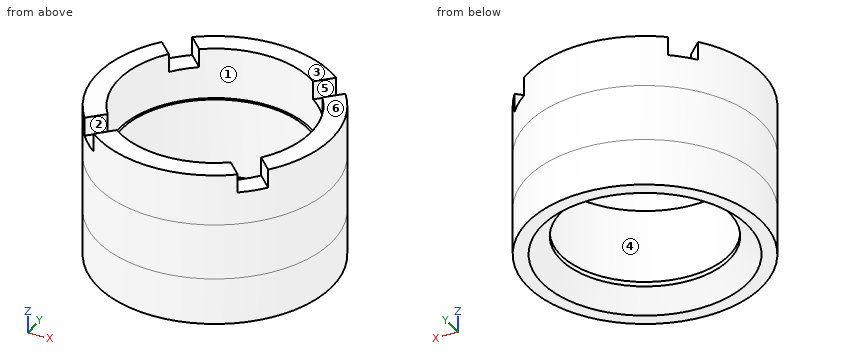
from build123d import *

# Parameters (mm, degrees)
F0_R      = 27
F0_R_2    = 18
F1_DEPTH  = 22
F2_R      = 20
F3_DEPTH  = 17
F4_SIZE   = 4
F5_R      = 27
F5_R_2    = 25
F6_DEPTH  = 12
F7_R      = 25
F7_R_2    = 20.5
F8_DEPTH  = 11
F10_DEPTH = 4
F11_R     = 27
F11_R_2   = 25
F12_DEPTH = 10.001


with BuildPart() as f1:
    # F0 (on Top) → F1 (new body)
    with BuildSketch(Plane.XY):
        Circle(F0_R)
        Circle(F0_R_2, mode=Mode.SUBTRACT)
    extrude(amount=-F1_DEPTH)

    # F2 (on face) → F3 (cut)
    with BuildSketch(Plane.XY):
        Circle(F2_R)
    extrude(amount=-F3_DEPTH, mode=Mode.SUBTRACT)

    # F4
    f4_edges = [f1.edges().sort_by_distance(p)[0] for p in [
        (-18, 0, -22),
    ]]
    chamfer(f4_edges, length=F4_SIZE)

    # F5 (on Top) → F6 (cut)
    with BuildSketch(Plane.XY):
        Circle(F5_R)
        Circle(F5_R_2, mode=Mode.SUBTRACT)
    extrude(amount=-F6_DEPTH, mode=Mode.SUBTRACT)

    # F7 (on face) → F8 (join)
    with BuildSketch(Plane.XY):
        Circle(F7_R)
        Circle(F7_R_2, mode=Mode.SUBTRACT)
    extrude(amount=F8_DEPTH)

    # F9 (on face) → F10 (cut)
    with BuildSketch(Plane.XY.offset(11)):
        Polygon((-28.467241, 32.709882), (-32.709882, 28.467241), (-4.242641, 0), (0, 4.242641), align=None)
        Polygon((0, -4.242641), (-4.242641, 0), (-34.573084, -30.330443), (-30.330443, -34.573084), align=None)
        Polygon((4.242641, 0), (0, -4.242641), (30.929728, -35.172369), (35.172369, -30.929728), align=None)
        Polygon((29.066526, 33.309167), (0, 4.242641), (4.242641, 0), (33.309167, 29.066526), align=None)
    extrude(amount=-F10_DEPTH, mode=Mode.SUBTRACT)

    # F11 (on face) → F12 (cut, through all)
    with BuildSketch(Plane.XY.offset(-12)):
        Circle(F11_R)
        Circle(F11_R_2, mode=Mode.SUBTRACT)
    extrude(amount=-F12_DEPTH, mode=Mode.SUBTRACT)


solid = f1.part
Geometry: final body of the model. Coordinates: model frame, mm. Face numbers are marked on the shaded views. A direction names the side the tool comes from. Round coordinates to 2 decimals unless told otherwise and drop trailing zeros. Order: outer loops, then holes, each group sorted by start corner. A loop starts at its lowest first (then second) coordinate and runs counter-clockwise, first axis right, second up.
Q1. Section D-D, the plane z = -6.5. Output: boundary loops of the cut face in (x, y).
Result sheet:
outline: circle Ø50 at (0, 0); hole circle Ø40 at (0, 0)
Q2. Section C-C, the plane z = 8. Output: boundary loops of the cut face in (x, y), and give its area (3 significant figures).
Result sheet:
outline: (-19.67, -15.43) - (-16.46, -12.22) arc R20.5 cw to (-16.46, 12.22) - (-19.67, 15.43) arc R25 ccw to start; (-15.43, -19.67) arc R25 ccw to (15.43, -19.67) - (12.22, -16.46) arc R20.5 cw to (-12.22, -16.46) - close; (-15.43, 19.67) - (-12.22, 16.46) arc R20.5 cw to (12.22, 16.46) - (15.43, 19.67) arc R25 ccw to start; (16.46, -12.22) - (19.67, -15.43) arc R25 ccw to (19.67, 15.43) - (16.46, 12.22) arc R20.5 cw to start
area: 535 mm2
Q3. Access query for the marked faces 1, 2 and 3. Directions: +Z, -Z, +X, -X, +Y, -Y. A direction counts if a zero-diameter tool reaches every point of the face in a straight line with its end or side. Return the directions, or none.
Result sheet:
face 1: +Z
face 2: +Z, -Y
face 3: +Z, +X, -X, +Y, -Y
Q4. Section A-A, the plane y = 0. Output: boundary loops of the cut face in (x, z), and give its area (3 significant figures).
Result sheet:
outline: (-25, -22) - (-22, -22) - (-18, -18) - (-18, -17) - (-20, -17) - (-20, 0) - (-20.5, 0) - (-20.5, 11) - (-25, 11) - close; (18, -18) - (22, -22) - (25, -22) - (25, 11) - (20.5, 11) - (20.5, 0) - (20, 0) - (20, -17) - (18, -17) - close
area: 323 mm2
Q5. Material intervals for probe 1 along X at (y, z) = (0, 8); probe 2 along Y at (x, z) = (0, -12); probe 3 along Y at (x, z) = (5, -1.5), sorted ascending.
Result sheet:
probe 1: x = -25 to -20.5, 20.5 to 25
probe 2: y = -25 to -20, 20 to 25
probe 3: y = -24.49 to -19.36, 19.36 to 24.49
Q6. Pin query (flat end, axial travel): pin 1 (5 mm diameter, centred on x = -13, z = 2, fed in from -Y); pin 2 (8 mm diameter, centred on x = -18, z = 5, fed in from -Y); pin 3 (1 mm diameter, centred on x = 14, z = 2.5, fed in from +Y). Return the tip coordinate at first contact, or that it passes through.
Result sheet:
pin 1: stops at y = -22.69
pin 2: stops at y = -20.71
pin 3: stops at y = 21.04
Q7. Mould query, pull axis X, two halves, no side actions, for the marked faces 4, 5 and 6. Classes: released by +X, released by -X, zero draft, split by the parting line, or undercut.
Result sheet:
face 4: undercut
face 5: released by +X
face 6: zero draft
